Geometry: final body of the model. Coordinates: model frame, mm. Face numbers are marked on the shaded views. A direction names the side the tool comes from. Coordinates: 2 decimals unless noted, no trailing zeros. Order: outer loops, then holes, each group sorted by start corner. A loop starts at its lowest first (then second) coordinate and runs counter-clockwise, first axis right, second up. Notation, with made-up numbers: (-7, 72) -> (49, 72) arc R11 ccw to (49, 89) -> close; hole circle Ø4 at (60.5, 27.25). An arc over 180 degrees is marked (long way). Answer in a Markdown table with one row per item. Add a question column.
1) Section query A-A on z = 0. Return the cut outline in (x, y).
2) Set-up query: the marked faces 1 and 2. Return all of +Z, -Z, +X, -X, +Y, -Y with unobstructed straight access to the full face (end or side cutting, diameter ignored); none if empty.
3) Section query D-D on z = -12.5. Return the cut outline in (x, y), then the cut area to 3 significant figures.
4) Section query B-B on y = 31.75. Return the cut outline in (x, z).
5) Ray query, line 1 (Y direction, x = 2, z = 0); line 2 (Z direction, x = 50.8, y = 4); line 3 (Y direction, x = 50, z = 21.5). Return the intervals inside material, ascending. Write a range as from..to.
6) Contact query for flat-ended pins moving along their axis: P1, Ø3, axis at x = 53, z = -18, coming from the +Y side; P2, Ø2, axis at y = 39, z = 18.5, coming from the -X side. Output: stop coordinate, or through.
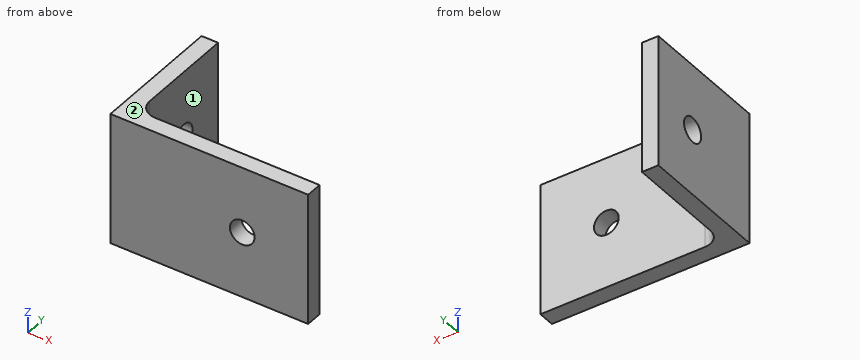
```python
from build123d import *

# Parameters (mm, degrees)
BRACKET_DEPTH      = 25.4
FILLET_2_R         = 6.35
SKETCH2_R          = 4.7625
BASE_HOLE_DEPTH    = 92.800885072
SKETCH4_R          = 4.7625
CUT_EXTRUDE2_DEPTH = 96.038097624


with BuildPart() as part:
    # Sketch1 → Bracket (new, symmetric)
    with BuildSketch(Plane.XY):
        Polygon((0, 0), (76.2, 0), (76.2, 6.35), (6.35, 6.35), (6.35, 50.8), (0, 50.8), align=None)
    extrude(amount=BRACKET_DEPTH, both=True)

    # Fillet 2
    fillet_2_edges = [part.edges().sort_by_distance(p)[0] for p in [
        (6.35, 6.35, 0),
    ]]
    fillet(fillet_2_edges, radius=FILLET_2_R)

    # Sketch2 → Base hole (cut, through all)
    with BuildSketch(Plane(origin=(0, 6.35, 0), x_dir=(1, 0, 0), z_dir=(0, 1, 0))):
        with Locations(Location((50.8, 0, 0), (0, 0, 180))):
            Circle(SKETCH2_R)
    extrude(amount=-BASE_HOLE_DEPTH, mode=Mode.SUBTRACT)

    # Sketch4 → Cut-Extrude2 (cut, through all)
    with BuildSketch(Plane.ZY):
        with Locations((0, 31.75)):
            Circle(SKETCH4_R)
    extrude(amount=-CUT_EXTRUDE2_DEPTH, mode=Mode.SUBTRACT)


solid = part.part
```
Result:
| question | item | result |
|---|---|---|
| 1 | outline | (0, 0) -> (46.04, 0) -> (46.04, 6.35) -> (12.7, 6.35) arc R6.35 cw to (6.35, 12.7) -> (6.35, 26.99) -> (0, 26.99) -> close; (0, 36.51) -> (6.35, 36.51) -> (6.35, 50.8) -> (0, 50.8) -> close; (55.56, 0) -> (76.2, 0) -> (76.2, 6.35) -> (55.56, 6.35) -> close |
| 2 | face 1 | +Z, -Z, +X, +Y |
| 2 | face 2 | +Z, +X, -X, +Y, -Y |
| 3 | outline | (0, 0) -> (76.2, 0) -> (76.2, 6.35) -> (12.7, 6.35) arc R6.35 cw to (6.35, 12.7) -> (6.35, 50.8) -> (0, 50.8) -> close |
| 3 | area | 775 mm2 |
| 4 | outline | (0, -25.4) -> (6.35, -25.4) -> (6.35, -4.76) -> (0, -4.76) -> close; (0, 4.76) -> (6.35, 4.76) -> (6.35, 25.4) -> (0, 25.4) -> close |
| 5 | line 1 | 0..26.99, 36.51..50.8 |
| 5 | line 2 | -25.4..-4.76, 4.76..25.4 |
| 5 | line 3 | 0..6.35 |
| 6 | P1 | y = 6.35 |
| 6 | P2 | x = 0 |
